from build123d import *

# Parameters (mm, degrees)
F1_DEPTH  = 40
F2_W      = 40
F2_H      = 40
F3_DEPTH  = 704
F4_W      = 1090
F4_H      = 40
F4_W_2    = 40
F4_H_2    = 640
F4_H_3    = 190
F5_DEPTH  = 40
F6_W      = 40
F6_H      = 5
F7_DEPTH  = 80
F8_R      = 9
F7_FACE_W = 80
F7_FACE_H = 40
F9_DEPTH  = 30
F11_W     = 40
F11_H     = 40
F12_DEPTH = 1090
F13_R     = 5
F14_DEPTH = 1170


with BuildPart() as f1:
    # F0 (on Front) → F1 (new body)
    with BuildSketch(Plane.XZ):
        Polygon((-585, 20), (-585, -20), (-545, -20), (545, -20), (585, -20), (585, 20), align=None)
        Polygon((-545, -20), (-585, -20), (-585, -850), (-545, -850), (-545, -660), (-545, -620), align=None)
        Polygon((585, -20), (545, -20), (545, -620), (545, -660), (545, -850), (585, -850), align=None)
    extrude(amount=F1_DEPTH)

    # F2 (on face) → F3 (join)
    with BuildSketch(Plane(origin=(0, 0, 0), x_dir=(-1, 0, 0), z_dir=(0, 1, 0))):
        with Locations((-565, 0)):
            Rectangle(F2_W, F2_H)
        with Locations((565, 0)):
            Rectangle(F2_W, F2_H)
        with Locations((-565, -640)):
            Rectangle(F2_W, F2_H)
        with Locations((565, -640)):
            Rectangle(F2_W, F2_H)
    extrude(amount=F3_DEPTH)

    # F4 (on face) → F5 (join)
    with BuildSketch(Plane(origin=(0, 704, 0), x_dir=(-1, 0, 0), z_dir=(0, 1, 0))):
        Polygon((-545, 20), (-585, 20), (-585, -850), (-545, -850), (-545, -660), (-545, -620), align=None)
        with Locations((0, -640)):
            Rectangle(F4_W, F4_H)
        with Locations((565, -640)):
            Rectangle(F4_W_2, F4_H)
        with Locations((565, -300)):
            Rectangle(F4_W_2, F4_H_2)
        with Locations((565, -755)):
            Rectangle(F4_W_2, F4_H_3)
    extrude(amount=F5_DEPTH)


with BuildPart() as f7:
    # F6 (on face) → F7 (new body)
    with BuildSketch(Plane(origin=(545, 0, 0), x_dir=(0, -1, 0), z_dir=(-1, 0, 0))):
        with Locations((20, -847.5)):
            Rectangle(F6_W, F6_H)
    extrude(amount=-F7_DEPTH)


with BuildPart() as f7b:
    # F6 (on face) → F7, piece 2 (new body)
    with BuildSketch(Plane(origin=(545, 0, 0), x_dir=(0, -1, 0), z_dir=(-1, 0, 0))):
        with Locations((-724, -847.5)):
            Rectangle(F6_W, F6_H)
    extrude(amount=-F7_DEPTH)


with BuildPart() as f9_tool:
    # F8 (on face) + F7_face (on face) → F9 (new body)
    with BuildSketch(Plane.XY.offset(-845)):
        with Locations((585, -20)):
            Circle(F8_R)
    with BuildSketch(Plane(origin=(585, -20, -845), x_dir=(1, 0, 0), z_dir=(0, 0, 1))):
        with Locations((0, 744)):
            Rectangle(F7_FACE_W, F7_FACE_H)
    extrude(amount=-F9_DEPTH)


with BuildPart() as f1_1:
    add(f1.part)

    # F9: cut by f9_tool
    add(f9_tool.part, mode=Mode.SUBTRACT)

    # F10: F7 across plane


with BuildPart() as f7_1:
    add(f7.part)

    # F9: cut by f9_tool
    add(f9_tool.part, mode=Mode.SUBTRACT)


with BuildPart() as f7b_1:
    add(f7b.part)

    # F9: cut by f9_tool
    add(f9_tool.part, mode=Mode.SUBTRACT)


with BuildPart() as f1_2:
    add(f1_1.part)
    add(f7_1.part.mirror(Plane.YZ))


    add(f7_1.part)  # F12 merges F7
    # F11 (on face) → F12 (join, through all)
    with BuildSketch(Plane.YZ.offset(-545)):
        with Locations((130, 0)):
            Rectangle(F11_W, F11_H)
    extrude(amount=F12_DEPTH)

    # F13 (on face) → F14 (cut, through all)
    with BuildSketch(Plane.YZ.offset(585)):
        with Locations((340, 0)):
            Circle(F13_R)
        with Locations((640, 0)):
            Circle(F13_R)
        with Locations((40, 0)):
            Circle(F13_R)
    extrude(amount=-F14_DEPTH, mode=Mode.SUBTRACT)


solid = f1_2.part
Source: CAD feature listing. Evaluate the final solid. Frame: model axes, mm. A direction names the side the tool comes from. Coordinates: 2 decimals unless noted, no trailing zeros. Loops run counter-clockwise (first coordinate to the right, second up) from the corner with the lowest first, then second, coordinate; pieces in that order, holes last. Notation, with made-up numbers: (61.5, 86.5) - (65.5, 86.5) arc R23 cw to (65.5, 115.5) - close; hole circle Ø1 at (72.5, 67). An arc over 180 degrees is marked (long way). One line per item, written item: value. Start each with the question number.
1. Mould query, pull axis Y, two halves, no side actions, for faces 1 (the flat face through (-605, -20, -845)), 2 (the flat face through (3, 744, -639)), 3 (the flat face through (-565, 0, -316)). Classes: pulls with the +Y half, pulls with the -Y half, needs draft (parallel to the pull), parting line crosses it, or undercut.
2. Ray query, L1, parallel to Z at x = -571.5, y = 340; L2, parallel to X at y = 146, z = -656; L3, parallel to Y at x = 585, z = -847.7. Return the intervals inside material, ascending.
3. Contact query for flat-ended pins moving along their axis: P1, Ø16, axis at y = 640, z = 0, coming from the +X side; P2, Ø12, axis at x = -198.5, z = -3.5, coming from the +Y side; P3, Ø8, axis at x = 402.5, z = -663, coming from the -Y side. Output: stop coordinate, or through.
4. Set-up query: faces 4 (the flat face through (46, 142, -20)), 5 (the flat face through (-8, 110, 0)), 6 (the flat face through (-565, 347, -660)), 7 (the flat face through (-545, 224, -621)), 8 (the flat face through (605, -20, -845)). Return all of +Z, -Z, +X, -X, +Y, -Y with unobstructed straight access to the full face (end or side cutting, diameter ignored); none if empty.
5. Section A-A (z = -35). Return the cut outline in (x, y).
6. Section C-C (x = -407). Return the cut outline in (y, z), and give its area (3 significant figures).
7. Section B-B (y = 587). Return the cut outline in (x, z).
Verdict:
1. face 1: needs draft
1. face 2: pulls with the +Y half
1. face 3: undercut
2. L1: z = -660 to -620, -20 to -5, 5 to 20
2. L2: x = -585 to -545, 545 to 585
2. L3: y = -40 to -29, -11 to 0
3. P1: stops at x = 585
3. P2: stops at y = 150
3. P3: stops at y = 704
4. face 4: +X, -X
4. face 5: +Z, -Z
4. face 6: -Z, +X, -X
4. face 7: -Z, -Y
4. face 8: +Z, +X, +Y, -Y
5. outline: (-585, -40) - (-545, -40) - (-545, 0) - (-585, 0) - close; (-585, 704) - (-545, 704) - (-545, 744) - (-585, 744) - close; (545, -40) - (585, -40) - (585, 0) - (545, 0) - close; (545, 704) - (585, 704) - (585, 744) - (545, 744) - close
6. outline: (-40, -20) - (0, -20) - (0, 20) - (-40, 20) - close; (110, -20) - (150, -20) - (150, 20) - (110, 20) - close; (704, -660) - (744, -660) - (744, -620) - (704, -620) - close
6. area: 4,800 mm2
7. outline: (-585, -660) - (-545, -660) - (-545, -620) - (-585, -620) - close; (-585, -20) - (-545, -20) - (-545, 20) - (-585, 20) - close; (545, -660) - (585, -660) - (585, -620) - (545, -620) - close; (545, -20) - (585, -20) - (585, 20) - (545, 20) - close
